Verification items for this drawing (mm, ordinates from the low corner). Coordinates: 2 decimals unless noted, no trailing zeros. Write each loop counter-clockwise with the first axis right and the second up, starting at its lowest first coordinate (ties: lowest second). Pieces come first, ordered by that corner, then holes. Notation, with made-up numbers: M 65.5,37 L 88.5,37 A8 ccw 88.5,48 Z; hole C 39.25,59 d5. An arc over 180 degrees is marked long. Answer as CSV lines item,"result". Start each with the question number.
1) Section check B-B (z = 39.5). Record the cut outline in (x, y).
2) Material ranges on L1, parallel to Z at x = 43, y = 1; L2, parallel to X at y = 2.5, z = 35.5; L3, parallel to Z at x = 25.5, y = 2.25, recorded low to high. Write a range as [from, to].
3) Section check D-D (x = 54). Record the cut outline in (y, z), and give its area (3 significant figures).
4) Section check A-A (x = 73). Record the cut outline in (y, z).
5) Section check C-C (y = 0.6). State how many separate pieces and enclosed holes the cut face has, and give its area (3 significant figures).
6) Go/stop test with flat-tipped pins: pin 1 Ø0.9 at (x, y) = (114.5, 1) entering from +Z; pin 2 Ø0.8 at (x, y) = (29.5, 1.5) entering from -Z; pin 3 Ø1.5 at (x, y) = (59, 1.5) entering from +Z. Record where each tip stops, or that it passes through.
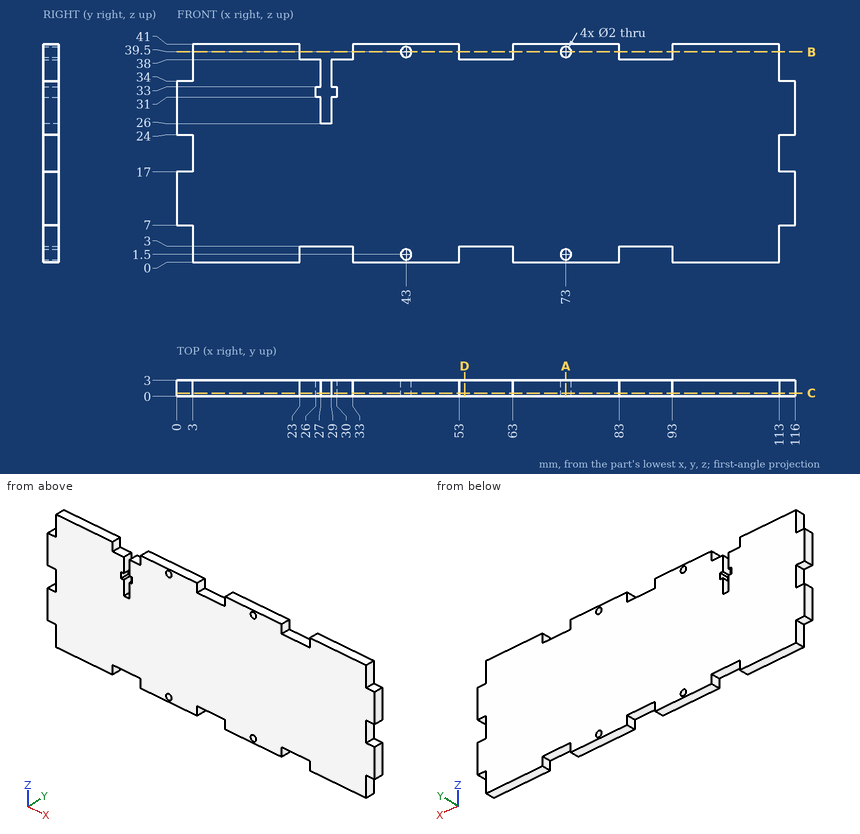
Results found:
1,outline,"M 3,0 L 23,0 L 23,3 L 3,3 Z; M 33,0 L 42,0 L 42,3 L 33,3 Z; M 44,0 L 53,0 L 53,3 L 44,3 Z; M 63,0 L 72,0 L 72,3 L 63,3 Z; M 74,0 L 83,0 L 83,3 L 74,3 Z; M 93,0 L 113,0 L 113,3 L 93,3 Z"
2,L1,"z = [0, 0.5], [2.5, 38.5], [40.5, 41]"
2,L2,"x = [3, 27], [29, 113]"
2,L3,"z = [3, 38]"
3,outline,"M 0,3 L 3,3 L 3,38 L 0,38 Z"
3,area,"105 mm2"
4,outline,"M 0,0 L 3,0 L 3,0.5 L 0,0.5 Z; M 0,2.5 L 3,2.5 L 3,38.5 L 0,38.5 Z; M 0,40.5 L 3,40.5 L 3,41 L 0,41 Z"
5,separate pieces,"1"
5,enclosed holes,"4"
5,area,"4,410 mm2"
6,pin 1,"stops at z = 34"
6,pin 2,"stops at z = 3"
6,pin 3,"stops at z = 38"
